The model under review builds one solid part; all positions refer to its coordinate system, in mm. A direction names the side the tool comes from. Coordinates: 2 decimals unless noted, no trailing zeros. Order: outer loops, then holes, each group sorted by start corner. A loop starts at its lowest first (then second) coordinate and runs counter-clockwise, first axis right, second up.
```python
from build123d import *

# Parameters (mm, degrees)
SKETCH1_W              = 398.11784
SKETCH1_H              = 394.318
SKETCH1_W_2            = 393.79984
SKETCH1_H_2            = 390
EXTRUDE_THIN1_DEPTH    = 375
CUT_EXTRUDE1_REACH     = 581.427
SKETCH2_W              = 318.11784
SKETCH2_H              = 375
CONVERT_SOLID1_START   = -375
CONVERT_SOLID1_DEPTH   = 375
CONVERT_SOLID1_2_DEPTH = 375


# Read off the part's stored shape, not the designer's step: Convert-Solid1
with BuildPart() as part:
    # Sketch1 → Extrude-Thin1 (new body)
    with BuildSketch(Plane(origin=(0, 0, 0), x_dir=(1, 0, 0), z_dir=(0, 1, 0))):
        Rectangle(SKETCH1_W, SKETCH1_H)
        Rectangle(SKETCH1_W_2, SKETCH1_H_2, mode=Mode.SUBTRACT)
    extrude(amount=-EXTRUDE_THIN1_DEPTH)

    # Sketch2 → Cut-Extrude1 (cut, up to next)
    with BuildSketch(Plane.XY.offset(197.159), mode=Mode.PRIVATE) as cut_extrude1_sk1:
        with Locations((0, -187.5)):
            Rectangle(SKETCH2_W, SKETCH2_H)
    cut_extrude1_tool1 = extrude(cut_extrude1_sk1.sketch, amount=-CUT_EXTRUDE1_REACH, mode=Mode.PRIVATE) & part.part
    add(cut_extrude1_tool1.solids().sort_by_distance((0, -187.5, 197.159))[0], mode=Mode.SUBTRACT)

    # Convert-Solid1 outline → Convert-Solid1 (cut)
    with BuildSketch(Plane(origin=(0, 0, 0), x_dir=(1, 0, 0), z_dir=(0, 1, 0)).offset(CONVERT_SOLID1_START)):
        with BuildLine():
            Line((199.05892, -197.159), (199.05892, -194.619))
            ThreePointArc((199.05892, -194.619), (198.314971224, -196.415051224), (196.51892, -197.159))
            Line((196.51892, -197.159), (199.05892, -197.159))
        make_face()
        with BuildLine():
            Line((199.05892, 197.159), (196.51892, 197.159))
            ThreePointArc((196.51892, 197.159), (198.314971224, 196.415051224), (199.05892, 194.619))
            Line((199.05892, 194.619), (199.05892, 197.159))
        make_face()
        with BuildLine():
            Line((-199.05892, 197.159), (-199.05892, 194.619))
            ThreePointArc((-199.05892, 194.619), (-198.314971224, 196.415051224), (-196.51892, 197.159))
            Line((-196.51892, 197.159), (-199.05892, 197.159))
        make_face()
        with BuildLine():
            ThreePointArc((-196.51892, -197.159), (-198.314971224, -196.415051224), (-199.05892, -194.619))
            Line((-199.05892, -194.619), (-199.05892, -197.159))
            Line((-199.05892, -197.159), (-196.51892, -197.159))
        make_face()
    extrude(amount=CONVERT_SOLID1_DEPTH, mode=Mode.SUBTRACT)

    # Convert-Solid1 2 outline → Convert-Solid1 2 (add)
    with BuildSketch(Plane(origin=(0, 0, 0), x_dir=(1, 0, 0), z_dir=(0, 1, 0)).offset(CONVERT_SOLID1_START)):
        with BuildLine():
            Line((196.89992, -195), (196.89992, -194.619))
            ThreePointArc((196.89992, -194.619), (196.788327684, -194.888407684), (196.51892, -195))
            Line((196.51892, -195), (196.89992, -195))
        make_face()
        with BuildLine():
            Line((196.89992, 195), (196.51892, 195))
            ThreePointArc((196.51892, 195), (196.788327684, 194.888407684), (196.89992, 194.619))
            Line((196.89992, 194.619), (196.89992, 195))
        make_face()
        with BuildLine():
            Line((-196.89992, 195), (-196.89992, 194.619))
            ThreePointArc((-196.89992, 194.619), (-196.788327684, 194.888407684), (-196.51892, 195))
            Line((-196.51892, 195), (-196.89992, 195))
        make_face()
        with BuildLine():
            ThreePointArc((-196.51892, -195), (-196.788327684, -194.888407684), (-196.89992, -194.619))
            Line((-196.89992, -194.619), (-196.89992, -195))
            Line((-196.89992, -195), (-196.51892, -195))
        make_face()
    extrude(amount=CONVERT_SOLID1_2_DEPTH)


solid = part.part
```
(1) Draft analysis for pull direction Z (two halves, no side actions). For faces 1 (the face through (-178, -185, 197.159)), 2 (the face through (-199.059, -185, 3)), 3 (the face through (178, -185, 195)), state which applies: released by +Z, released by -Z, zero draft, split by the parting line, or undercut.
A:
face 1: released by +Z
face 2: zero draft
face 3: undercut
(2) Wall thickness on probe 1 along X at (y, z) = (-304.5, 15); probe 2 along Z at (x, y) = (-81, -54); probe 3 along Z at (x, y) = (-162.5, -133.5): over which ranges is each line inside the solid? List them lowest first.
A:
probe 1: x = -199.06 to -196.9, 196.9 to 199.06
probe 2: z = -197.16 to -195
probe 3: z = -197.16 to -195, 195 to 197.16
(3) We need section C-C, the plane y = -320. Write out the cut boundary in (x, z).
A:
outline: (-199.06, -194.62) arc R2.54 ccw to (-196.52, -197.16) - (196.52, -197.16) arc R2.54 ccw to (199.06, -194.62) - (199.06, 194.62) arc R2.54 ccw to (196.52, 197.16) - (159.06, 197.16) - (159.06, 195) - (196.52, 195) arc R0.38 cw to (196.9, 194.62) - (196.9, -194.62) arc R0.38 cw to (196.52, -195) - (-196.52, -195) arc R0.38 cw to (-196.9, -194.62) - (-196.9, 194.62) arc R0.38 cw to (-196.52, 195) - (-159.06, 195) - (-159.06, 197.16) - (-196.52, 197.16) arc R2.54 ccw to (-199.06, 194.62) - close
(4) We need section B-B, the plane z = 29.5. Write out the cut boundary in (x, y), and give its area (3 significant figures).
A:
outline: (-199.06, -375) - (-196.9, -375) - (-196.9, 0) - (-199.06, 0) - close; (196.9, -375) - (199.06, -375) - (199.06, 0) - (196.9, 0) - close
area: 1,620 mm2
(5) We need section D-D, the plane x = 121. Write out the cut boundary in (y, z), and give its area (3 significant figures).
A:
outline: (-375, -197.16) - (0, -197.16) - (0, -195) - (-375, -195) - close
area: 810 mm2
(6) For pin 1 Ø2 at (x, y) = (-52.5, -187) entering from +Z; pin 2 Ø1.7 at (y, z) = (-203.5, 196.5) entering from -X; pin 3 Ø2.5 at (y, z) = (-145.5, 196.5) entering from +X, all flat-tipped, find the tip position at first contact; note any pin that passes through.
A:
pin 1: stops at z = -195
pin 2: stops at x = -198.84
pin 3: stops at x = 198.98
(7) We need section A-A, the plane x = -171. Write out the cut boundary in (y, z).
A:
outline: (-375, -197.16) - (0, -197.16) - (0, -195) - (-375, -195) - close; (-375, 195) - (0, 195) - (0, 197.16) - (-375, 197.16) - close
(8) Machinability: for faces 4 (the face through (178, -185, 197.159)), 5 (the face through (196.9, -185, 3)), which of the approach directions +Z, -Z, +X, -X, +Y, -Y give a long, thin tool a straight path to every point of the face, cutting with its end or side? Answer none if there is none.
A:
face 4: +Z, +X, -X, +Y, -Y
face 5: +Y, -Y
